Input: part model. Units: mm. Frame: model coordinates. Face numbers are marked on the shaded views. A direction names the side the tool comes from. Coordinates: 2 decimals unless noted, no trailing zeros. Order: outer loops, then holes, each group sorted by start corner. A loop starts at its lowest first (then second) coordinate and runs counter-clockwise, first axis right, second up. Notation, with made-up numbers: (45, 19) -> (75, 19) arc R18 cw to (75, 43) -> close; hole circle Ø3 at (81.25, -21). An arc over 180 degrees is marked (long way). One line per item, written item: value. Start each with the question number.
from build123d import *

# Parameters (mm, degrees)
F0_W      = 86.565242
F0_H      = 62.221606
F1_DEPTH  = 76.2
F2_R      = 9.525
F1_FACE_W = 76.2
F1_FACE_H = 52.696606
F3_DEPTH  = 25.4


with BuildPart() as f1:
    # F0 (on Front) → F1 (new body)
    with BuildSketch(Plane.XZ):
        Rectangle(F0_W, F0_H)
    extrude(amount=F1_DEPTH)

    # F2
    f2_edges = [f1.edges().sort_by_distance(p)[0] for p in [
        (43.282621, -38.1, 31.110803),
    ]]
    fillet(f2_edges, radius=F2_R)

    # F1_face (on face) → F3 (join)
    with BuildSketch(Plane(origin=(43.282621, -38.1, -4.7625), x_dir=(0, 1, 0), z_dir=(1, 0, 0))):
        Rectangle(F1_FACE_W, F1_FACE_H)
    extrude(amount=F3_DEPTH)


solid = f1.part
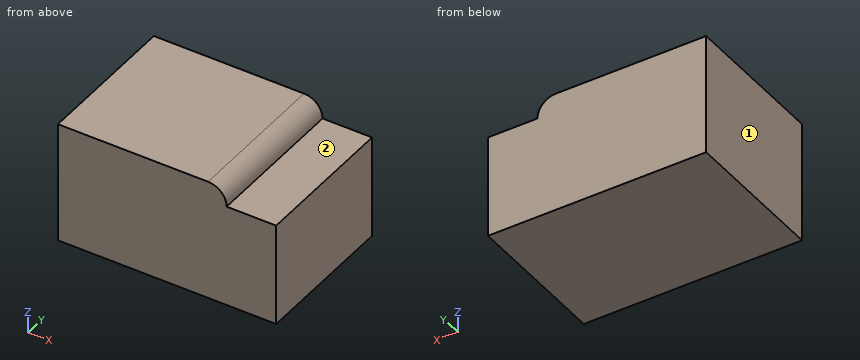
1) Ray query, line 1 along Z through (x, y) = (50, -3.5); line 2 along Z through (x, y) = (38.5, -23.5). Return the intervals inside material, ascending. Write a range as from..to.
2) Access query for the marked faces 1 and 2. Directions: +Z, -Z, +X, -X, +Y, -Y. A direction counts if a zero-diameter tool reaches every point of the face in a straight line with its end or side. Return the directions, or none.
3) Section query A-A, the plane y = -68.5. Return the cut outline in (x, z) (3 decimals).
4) Section query B-B, the plane x = 46.5. Return the cut outline in (y, z).
5) Section query C-C, the plane z = 26.5. Return the cut outline in (x, y), plus the area to 3 significant figures.
6) Pin query (flat end, axial travel): pin 1 Ø12.5 at (x, y) = (59, -21.5) entering from +Z. Return the tip coordinate at first contact, or that it passes through.
Entries:
1. line 1: z = -31.11..21.59
1. line 2: z = -31.11..29.85
2. face 1: +Z, -Z, -X, +Y, -Y
2. face 2: +Z, +X, +Y, -Y
3. outline: (-43.283, -31.111) -> (68.683, -31.111) -> (68.683, 21.586) -> (43.283, 21.586) arc R9.525 ccw to (33.758, 31.111) -> (-43.283, 31.111) -> close
4. outline: (-76.2, -31.11) -> (0, -31.11) -> (0, 21.59) -> (-76.2, 21.59) -> close
5. outline: (-43.28, -76.2) -> (41.92, -76.2) -> (41.92, 0) -> (-43.28, 0) -> close
5. area: 6,490 mm2
6. pin 1: stops at z = 21.59
